```python
from build123d import *

# Parameters (mm, degrees)
ESQUISSE1_W        = 3
ESQUISSE1_H        = 2
BOSS_EXTRU_1_DEPTH = 3
CONG_1_R           = 1
CONG_3_R           = 0.5
ESQUISSE4_W        = 0.9
ESQUISSE4_H        = 6.05


with BuildPart() as part:
    # Esquisse1 → Révolution1 (revolve)
    with BuildSketch(Plane.XY):
        with Locations((1.5, 5.05)):
            Rectangle(ESQUISSE1_W, ESQUISSE1_H)
    revolve(axis=Axis((-3.996004355, 0, 0), (1, 0, 0)))

    # Esquisse2 → Boss.-Extru.1 (add)
    with BuildSketch(Plane.ZY):
        with BuildLine():
            Line((5.958086906, -1.050571475), (8.420106288, -1.484691919))
            ThreePointArc((8.420106288, -1.484691919), (8.55, 0), (8.420106288, 1.484691919))
            Line((8.420106288, 1.484691919), (5.958086906, 1.050571475))
            ThreePointArc((5.958086906, 1.050571475), (6.05, 0), (5.958086906, -1.050571475))
        make_face()
    extrude(amount=-BOSS_EXTRU_1_DEPTH)

    # Congé1
    cong_1_edges = [part.edges().sort_by_distance(p)[0] for p in [
        (1.5, -1.050571475, 5.958086906),
        (1.5, 1.050571475, 5.958086906),
    ]]
    fillet(cong_1_edges, radius=CONG_1_R)

    # Congé3
    cong_3_edges = [part.edges().sort_by_distance(p)[0] for p in [
        (1.5, 1.484691919, 8.420106288),
        (1.5, -1.484691919, 8.420106288),
    ]]
    fillet(cong_3_edges, radius=CONG_3_R)

    # Esquisse4 → Dégagement M21 (revolve, cut)
    with BuildSketch(Plane(origin=(1.5, 0, 0), x_dir=(0, -1, 0), z_dir=(1, 0, 0))):
        with Locations((0.45, 3.025)):
            Rectangle(ESQUISSE4_W, ESQUISSE4_H)
    revolve(axis=Axis((1.5, 0, 6.35), (0, 0, -1)), mode=Mode.SUBTRACT)


solid = part.part
```
Part model, mm, in its own coordinate system. A direction names the side the tool comes from. Round coordinates to 2 decimals unless told otherwise and drop trailing zeros. Loops run counter-clockwise (first coordinate to the right, second up) from the corner with the lowest first, then second, coordinate; pieces in that order, holes last. Notation, with made-up numbers: (-35.5, -1.75) -> (-13.5, -1.75) arc R13 ccw to (-13.5, 6.25) -> close; hole circle Ø5 at (68.25, 46.5). An arc over 180 degrees is marked (long way). Use one line per item in the form item = value. Start each with the question number.
Item 1: Two-plate mould, pull along X, no slides. Class faces 1 (the flat face through (1.479, 1.305, 7.4)), 2 (the cylindrical face through (0.61, 0.12, -5.01)), 3 (the flat face through (3, 3, 3)): released by +X, released by -X, zero draft, split by the parting line, or undercut.
Item 2: Tool access for faces 4 (the cylindrical face through (1.48, -0.01, 8.55)), 5 (the flat face through (1.479, -1.302, 7.385)): list every direction of +Z, -Z, +X, -X, +Y, -Y with a clear straight run to the whole face (end or side of a thin tool).
Item 3: Band-saw the part on B-B (y = 0). List the corners of the cut face in (x, z).
Item 4: Drill centre lines: line 1 along X through (y, z) = (0, -5); line 2 along Z through (x, y) = (0.9, 0); line 3 along Z through (x, y) = (2.25, 3). Where is each one in solid material? Low to high.
Item 5: Band-saw the part on D-D (y = 2.25). List the corners of the cut face in (x, z), plus the area to 3 significant figures.
Item 6: Band-saw the part on A-A (z = 0). List the corners of the cut face in (x, y), plus the area to 3 significant figures.
Item 7: Band-saw the part on C-C (x = 0.35). List the corners of the cut face in (y, z), plus the area to 3 significant figures.
Item 8: Drop flat-ended pins along their axis: pin 1 Ø1 at (x, y) = (1.5, 3) entering from -Z; pin 2 Ø3 at (y, z) = (-2, 0) entering from +X; pin 3 Ø1.4 at (x, y) = (1.5, 0) entering from -Z. Give the stop position or say it passes through.
Data:
q1.face_1 = zero draft
q1.face_2 = undercut
q1.face_3 = released by +X
q2.face_4 = +Z, +X, -X
q2.face_5 = +X, -X, -Y
q3.outline = (0, -6.05) -> (0.6, -6.05) -> (0.6, -4.05) -> (0, -4.05) -> close; (0, 4.05) -> (3, 4.05) -> (3, 8.55) -> (0, 8.55) -> close; (2.4, -6.05) -> (3, -6.05) -> (3, -4.05) -> (2.4, -4.05) -> close
q4.line_1 = 0 to 0.6, 2.4 to 3
q4.line_2 = 4.05 to 8.55
q4.line_3 = -5.25 to -2.72, 2.72 to 5.25
q5.outline = (0, -5.62) -> (3, -5.62) -> (3, -3.37) -> (0, -3.37) -> close; (0, 3.37) -> (3, 3.37) -> (3, 5.62) -> (0, 5.62) -> close
q5.area = 13.5 mm^2
q6.outline = (0, -6.05) -> (3, -6.05) -> (3, -4.05) -> (0, -4.05) -> close; (0, 4.05) -> (3, 4.05) -> (3, 6.05) -> (0, 6.05) -> close
q6.area = 12.0 mm^2
q7.outline = (-1.89, 5.75) arc R6.05 ccw (long way) to (1.89, 5.75) arc R1 cw to (1.21, 6.87) -> (1.4, 7.91) arc R0.5 ccw to (0.96, 8.5) arc R8.55 ccw to (-0.96, 8.5) arc R0.5 ccw to (-1.4, 7.91) -> (-1.21, 6.87) arc R1 cw to start; hole circle Ø8.1 at (0, 0)
q7.area = 70.1 mm^2
q8.pin_1 = -5.51
q8.pin_2 = through
q8.pin_3 = 3.99
